from build123d import *

# Parameters (mm, degrees)
F0_R     = 6.746875
F1_DEPTH = 1.190625
F2_R     = 5.953125
F3_DEPTH = 3.571875
F4_R     = 0.396875
F5_R     = 0.198437
F6_R     = 5.55625
F7_DEPTH = 2.38125
F8_W     = 6.35
F8_H     = 6.35
F9_DEPTH = 0.396875


with BuildPart() as f1:
    # F0 (on Front) → F1 (new body)
    with BuildSketch(Plane.XZ):
        Circle(F0_R)
    extrude(amount=-F1_DEPTH)

    # F2 (on face) → F3 (join)
    with BuildSketch(Plane(origin=(0, 1.190625, 0), x_dir=(-1, 0, 0), z_dir=(0, 1, 0))):
        Circle(F2_R)
    extrude(amount=F3_DEPTH)

    # F4
    f4_edges = [f1.edges().sort_by_distance(p)[0] for p in [
        (5.953125, 4.7625, 0),
    ]]
    fillet(f4_edges, radius=F4_R)

    # F5
    f5_edges = [f1.edges().sort_by_distance(p)[0] for p in [
        (5.953125, 1.190625, 0),
        (-6.746875, 1.190625, 0),
    ]]
    fillet(f5_edges, radius=F5_R)

    # F6 (on face) → F7 (cut)
    with BuildSketch(Plane(origin=(0, 4.7625, 0), x_dir=(-1, 0, 0), z_dir=(0, 1, 0))):
        Circle(F6_R)
    extrude(amount=-F7_DEPTH, mode=Mode.SUBTRACT)

    # F8 (on face) → F9 (join)
    with BuildSketch(Plane(origin=(0, 2.38125, 0), x_dir=(-1, 0, 0), z_dir=(0, 1, 0))):
        Rectangle(F8_W, F8_H)
    extrude(amount=F9_DEPTH)


solid = f1.part
For this review, take the finished solid that the model builds, in its own axes (mm). A direction names the side the tool comes from. Give positions to 0.01 mm unless a question says otherwise; leave off trailing zeros. Loops run counter-clockwise (first coordinate to the right, second up) from the corner with the lowest first, then second, coordinate; pieces in that order, holes last. Notation, with made-up numbers: M -8,-14.75 L 38,-14.75 A11 cw 38,5.25 Z; hole C -2.5,40 d3. An arc over 180 degrees is marked long. Answer as a JSON object with one key per item and string values. Group by question number.
Q1. Mouldability with a two-part tool opening along X and no side actions: class faces 3 (the cylindrical face through (4.724, 2.857, -3.622)), 4 (the flat face through (0, 0, 0)), 5 (the cylindrical face through (-5.3, 3.59, 1.67)) as +X half, -X half, draft (parallel to the pull), parting line (faces both ways), or undercut.
Q2. Add section D-D on y = 1.55. Give the boundary of the cut face in (x, z).
Q3. Insertion check: P1, Ø1, axis at y = 3.5, z = 2, coming from the -X side; P2, Ø1.9, axis at x = 0.5, z = -0.5, coming from the +Y side. Each pin has a flat end and moves straight along its axis. Give the tip position at first contact, or say it passes through.
Q4. Tool access review of faces 1 (the flat face through (0, 2.778, 0)), 2 (the cylindrical face through (-4.97, 0.49, 4.56)): name each direction out of +Z, -Z, +X, -X, +Y, -Y from which nothing blocks a thin tool from reaching the whole face with its end or side.
Q5. Add section B-B on y = 4.2. Give the boundary of the cut face in (x, z).
Q6. For probe 1 along Z at (x, y) = (0, 3.25); probe 2 along Y at (x, z) = (0.25, -1.5); probe 3 along Y at (x, z) = (-3.75, 3), list the stretches that pass through material, from the lowest coordinate up. Write a range as [from, to].
Checked values:
{
 "1": {"face 3": "parting line", "face 4": "draft", "face 5": "undercut"},
 "2": {"outline": "C 0,0 d11.91"},
 "3": {"P1": "x = -5.76", "P2": "y = 2.78"},
 "4": {"face 1": "+Y", "face 2": "+Y, -Y"},
 "5": {"outline": "C 0,0 d11.91; hole C 0,0 d11.11"},
 "6": {"probe 1": "[-5.95, -5.56], [5.56, 5.95]", "probe 2": "[0, 2.78]", "probe 3": "[0, 2.38]"}
}
